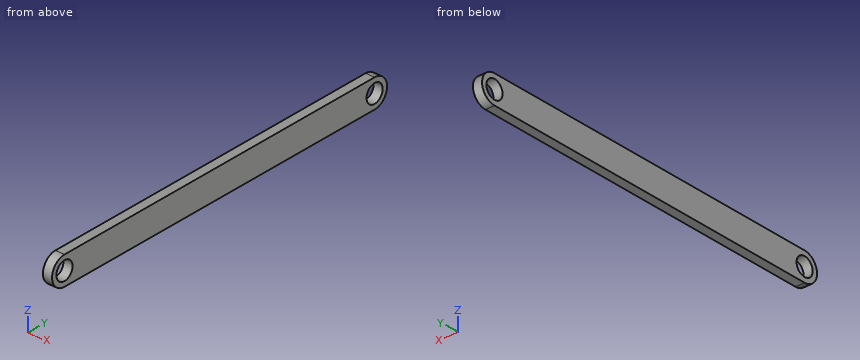
Autodesk Inventor part; units mm, degrees
ref_plane "YZ Plane" through (0, 0, 0) normal (1, 0, 0) x (0, 1, 0)
ref_plane "XZ Plane" through (0, 0, 0) normal (0, 1, 0) x (-1, 0, 0)
ref_plane "XY Plane" through (0, 0, 0) normal (0, 0, 1) x (1, 0, 0)
sketch "Sketch1" plane through (0, 0, 0) normal (1, 0, 0) x (0, 1, 0)
  circle A0 centre (0, 0) radius 6.35
  arc A1 (0, 9.779) -> (0, -9.779) centre (0, 0) ccw
  line L0 (0, 9.779) -> (244.2972, 9.779)
  line L1 (0, -9.779) -> (244.2972, -9.779)
  arc A2 (244.2972, -9.779) -> (244.2972, 9.779) centre (244.2972, 0) ccw
  circle A3 centre (244.2972, 0) radius 6.35
  dimension "d0" = 12.7
  dimension "d1" = 19.558
  dimension "d2" = 244.2972
  dimension "d3" = 244.2972
  dimension "d4" = 12.7
extrude "Extrusion1" add sketch "Sketch1" along normal blind 6.35
properties part number "RollerArm"
Verification items for the finished model (mm, model axes). Give positions to 0.01 mm unless a question says otherwise; leave off trailing zeros. Order: outer loops, then holes, each group sorted by start corner. A loop starts at its lowest first (then second) coordinate and runs counter-clockwise, first axis right, second up. Notation, with made-up numbers: (-5, 73) -> (23, 73) arc R12 cw to (23, 83) -> close; hole circle Ø4 at (65.5, 54.5). An arc over 180 degrees is marked (long way). Use a Markdown table: item, result.
1) Material ranges on probe 1 along Y at (x, z) = (4.5, 0.25); probe 2 along Y at (x, z) = (3, -0.75); probe 3 along Y at (x, z) = (1.25, 8.5), recorded low to high.
Results:
| item | result |
|---|---|
| probe 1 | -9.78 to -6.35, 6.35 to 237.95, 250.64 to 254.07 |
| probe 2 | -9.75 to -6.31, 6.31 to 237.99, 250.6 to 254.05 |
| probe 3 | -4.84 to 249.13 |
2) Section check B-B, the plane x = 4.75. Record the boundary of the cut face in (y, z), then the cut area to 3 significant figures.
Results:
| item | result |
|---|---|
| outline | (0, -9.78) -> (244.3, -9.78) arc R9.78 ccw to (244.3, 9.78) -> (0, 9.78) arc R9.78 ccw to start; hole circle Ø12.7 at (0, 0); hole circle Ø12.7 at (244.3, 0) |
| area | 4,830 mm² |
3) Section check A-A, the plane z = 0. Record the boundary of the cut face in (x, y).
Results:
| item | result |
|---|---|
| outline | (0, -9.78) -> (6.35, -9.78) -> (6.35, -6.35) -> (0, -6.35) -> close; (0, 6.35) -> (6.35, 6.35) -> (6.35, 237.95) -> (0, 237.95) -> close; (0, 250.65) -> (6.35, 250.65) -> (6.35, 254.08) -> (0, 254.08) -> close |
4) Depth check by flat-ended pin: pin 1 Ø1 at (y, z) = (17, -6) entering from -X; pin 2 Ø2 at (x, z) = (2.5, -7.5) entering from -Y; pin 3 Ø3 at (x, z) = (1.5, 6) entering from +Y. Enter the tip coordinate at first touch or a pass-through.
Results:
| item | result |
|---|---|
| pin 1 | x = 0 |
| pin 2 | y = -7.31 |
| pin 3 | y = 252.98 |
